Can you work these out from the drawing? Everything is in mm from the part's minimum corner. A direction names the side the tool comes from. Round coordinates to 2 decimals unless told otherwise and drop trailing zeros. Loops run counter-clockwise (first coordinate to the right, second up) from the corner with the lowest first, then second, coordinate; pieces in that order, holes last. Notation, with made-up numbers: M 48.5,-5.5 L 81.5,-5.5 A18 cw 81.5,27.5 Z; hole C 75.5,-17.5 d1. An arc over 180 degrees is marked long. Use a Markdown table: item, result.
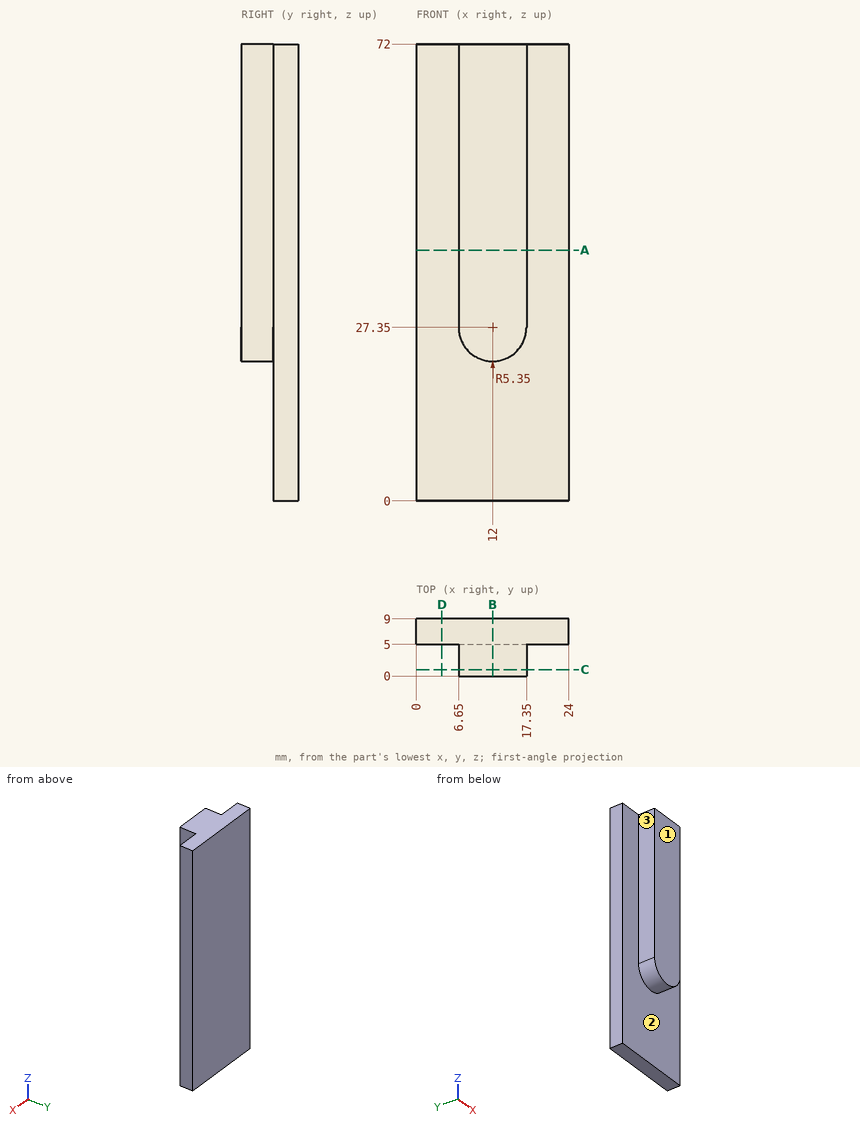
Q1. I need wall thicknesses on line 1 (Z direction, x = 12, y = 3.5); line 2 (Y direction, x = 8.5, z = 8); line 3 (X direction, y = 0.75, z = 60). Which ranges of each line are inside material? Lowest first, please. Write a range as from..to.
Return value:
| item | result |
|---|---|
| line 1 | z = 22..72 |
| line 2 | y = 5..9 |
| line 3 | x = 6.65..17.35 |
Q2. Imagine slicing it at C-C, the plane y = 1. Please give me the cut outline in (x, z).
Return value:
| item | result |
|---|---|
| outline | M 6.65,27.35 A5.35 ccw 17.35,27.35 L 17.35,72 L 6.65,72 Z |
Q3. For the marked faces 1, 2 and 3, which set-ups out of +Z, -Z, +X, -X, +Y, -Y let a thin tool reach every point of the face, with its end or its side?
Return value:
| item | result |
|---|---|
| face 1 | +Z, -Z, +X, -X, -Y |
| face 2 | -Z, -Y |
| face 3 | +Z, -Z, -X, -Y |
Q4. Will these pins go through, and if not, where does the flat tip stop? P1, Ø1, axis at y = 2, z = 42.5, coming from the -X side; P2, Ø2, axis at y = 6.5, z = 13, coming from the -X side; P3, Ø6, axis at x = 6.5, z = 21, coming from the -Y side; P4, Ø1.5, axis at y = 3, z = 60.5, coming from the +X side.
Return value:
| item | result |
|---|---|
| P1 | stops at x = 6.65 |
| P2 | stops at x = 0 |
| P3 | stops at y = 5 |
| P4 | stops at x = 17.35 |
Q5. Imagine slicing it at B-B, the plane x = 12. Please give me the cut outline in (y, z).
Return value:
| item | result |
|---|---|
| outline | M 0,22 L 5,22 L 5,0 L 9,0 L 9,72 L 0,72 Z |
Q6. Imagine slicing it at D-D, the plane x = 4. Please give me the cut outline in (y, z), then the cut area to 3 significant figures.
Return value:
| item | result |
|---|---|
| outline | M 5,0 L 9,0 L 9,72 L 5,72 Z |
| area | 288 mm^2 |
Q7. Imagine slicing it at A-A, the plane z = 39.5. Please give me the cut outline in (x, y).
Return value:
| item | result |
|---|---|
| outline | M 0,5 L 6.65,5 L 6.65,0 L 17.35,0 L 17.35,5 L 24,5 L 24,9 L 0,9 Z |
